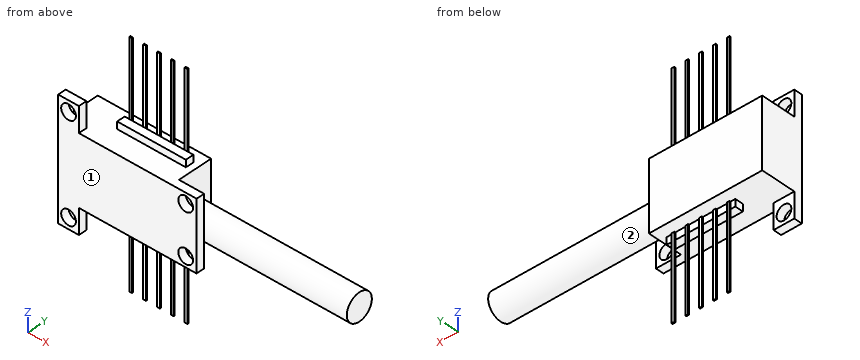
```python
from build123d import *

# Parameters (mm, degrees)
SKETCH1_W               = 20.8
SKETCH1_H               = 12.7
BOSS_EXTRUDE1_DEPTH     = 6.4
BOSS_EXTRUDE2_DEPTH     = 1.5
SKETCH5_R               = 1.35
CUT_EXTRUDE1_DEPTH      = 21.181984541
SKETCH8_R               = 2.5
BOSS_EXTRUDE3_DEPTH     = 30.15
SKETCH9_W               = 12.6
SKETCH9_H               = 1.3
BOSS_EXTRUDE4_DEPTH     = 1.5
SKETCH10_W              = 0.5
SKETCH10_H              = 15.3
BOSS_EXTRUDE5_DEPTH     = 0.2
LPATTERN1_COUNT         = 5
LPATTERN1_PITCH         = 2.54
MIRROR2_COPY_1_SKETCH_W = 0.5
MIRROR2_COPY_1_SKETCH_H = 15.3
MIRROR2_COPY_1_DEPTH    = 0.2
MIRROR2_COPY_2_SKETCH_W = 0.5
MIRROR2_COPY_2_SKETCH_H = 15.3
MIRROR2_COPY_2_DEPTH    = 0.2
MIRROR2_COPY_3_SKETCH_W = 0.5
MIRROR2_COPY_3_SKETCH_H = 15.3
MIRROR2_COPY_3_DEPTH    = 0.2
MIRROR2_COPY_4_SKETCH_W = 0.5
MIRROR2_COPY_4_SKETCH_H = 15.3
MIRROR2_COPY_4_DEPTH    = 0.2


with BuildPart() as part:
    # Sketch1 → Boss-Extrude1 (new body)
    with BuildSketch(Plane(origin=(0, 0, 0), x_dir=(1, 0, 0), z_dir=(0, 1, 0))):
        Rectangle(SKETCH1_W, SKETCH1_H)
    extrude(amount=BOSS_EXTRUDE1_DEPTH)

    # Sketch3 → Boss-Extrude2 (add)
    with BuildSketch(Plane.XZ):
        Polygon((-10.4, 10.95), (-6.6, 10.95), (-6.6, 6.35), (15, 6.35), (15, -6.35), (-6.6, -6.35), (-6.6, -10.95), (-10.4, -10.95), align=None)
    extrude(amount=BOSS_EXTRUDE2_DEPTH)

    # Sketch5 → Cut-Extrude1 (cut, through all)
    with BuildSketch(Plane.XZ.offset(1.5)):
        with Locations(Location((-8.5, 8.95, 0), (0, 0, 270))):
            Circle(SKETCH5_R)
        with Locations(Location((13, 4.45, 0), (0, 0, 270))):
            Circle(SKETCH5_R)
    cut_extrude1 = extrude(amount=-CUT_EXTRUDE1_DEPTH, mode=Mode.SUBTRACT)

    # Mirror3: Cut-Extrude1 across plane
    add(cut_extrude1.mirror(Plane.XY), mode=Mode.SUBTRACT)

    # Sketch8 → Boss-Extrude3 (add)
    with BuildSketch(Plane(origin=(10.4, 0, 0), x_dir=(0, 0, -1), z_dir=(1, 0, 0))):
        with Locations(Location((1.5, 3.2, 0), (0, 0, 180))):
            Circle(SKETCH8_R)
    extrude(amount=BOSS_EXTRUDE3_DEPTH)

    # Sketch9 → Boss-Extrude4 (add)
    with BuildSketch(Plane(origin=(0, 2.665, 0), x_dir=(-1, 0, 0), z_dir=(0, -1, 0))):
        with Locations((-2.9, -7)):
            Rectangle(SKETCH9_W, SKETCH9_H)
    boss_extrude4 = extrude(amount=-BOSS_EXTRUDE4_DEPTH)

    # Sketch10 → Boss-Extrude5 (add)
    with BuildSketch(Plane(origin=(0, 4.165, 0), x_dir=(1, 0, 0), z_dir=(0, 1, 0))):
        with Locations((7.87, -14)):
            Rectangle(SKETCH10_W, SKETCH10_H)
    boss_extrude5 = extrude(amount=BOSS_EXTRUDE5_DEPTH)

    # LPattern1: Boss-Extrude5 ×5
    with Locations(*[(-i * LPATTERN1_PITCH, 0, 0) for i in range(1, LPATTERN1_COUNT)]):
        add(boss_extrude5)

    # Mirror2: Boss-Extrude4, Boss-Extrude5 across plane
    add(boss_extrude4.mirror(Plane.XY))
    add(boss_extrude5.mirror(Plane.XY))

    # Mirror2 copy 1 sketch → Mirror2 copy 1 (add)
    with BuildSketch(Plane(origin=(-2.54, 4.165, 0), x_dir=(1, 0, 0), z_dir=(0, 1, 0))):
        with Locations((7.87, 14)):
            Rectangle(MIRROR2_COPY_1_SKETCH_W, MIRROR2_COPY_1_SKETCH_H)
    extrude(amount=MIRROR2_COPY_1_DEPTH)

    # Mirror2 copy 2 sketch → Mirror2 copy 2 (add)
    with BuildSketch(Plane(origin=(-5.08, 4.165, 0), x_dir=(1, 0, 0), z_dir=(0, 1, 0))):
        with Locations((7.87, 14)):
            Rectangle(MIRROR2_COPY_2_SKETCH_W, MIRROR2_COPY_2_SKETCH_H)
    extrude(amount=MIRROR2_COPY_2_DEPTH)

    # Mirror2 copy 3 sketch → Mirror2 copy 3 (add)
    with BuildSketch(Plane(origin=(-7.62, 4.165, 0), x_dir=(1, 0, 0), z_dir=(0, 1, 0))):
        with Locations((7.87, 14)):
            Rectangle(MIRROR2_COPY_3_SKETCH_W, MIRROR2_COPY_3_SKETCH_H)
    extrude(amount=MIRROR2_COPY_3_DEPTH)

    # Mirror2 copy 4 sketch → Mirror2 copy 4 (add)
    with BuildSketch(Plane(origin=(-10.16, 4.165, 0), x_dir=(1, 0, 0), z_dir=(0, 1, 0))):
        with Locations((7.87, 14)):
            Rectangle(MIRROR2_COPY_4_SKETCH_W, MIRROR2_COPY_4_SKETCH_H)
    extrude(amount=MIRROR2_COPY_4_DEPTH)


solid = part.part
```
Geometry: final body of the model. Coordinates: model frame, mm. Face numbers are marked on the shaded views. A direction names the side the tool comes from. Give positions to 0.01 mm unless a question says otherwise; leave off trailing zeros. Loops run counter-clockwise (first coordinate to the right, second up) from the corner with the lowest first, then second, coordinate; pieces in that order, holes last. Notation, with made-up numbers: (66, 74.25) -> (81, 74.25) arc R35 ccw to (81, 108.25) -> close; hole circle Ø5 at (46.5, -2.75). An arc over 180 degrees is marked (long way). Use one line per item in the form item = value.
Item 1: Section query D-D on x = -8.5. Output: boundary loops of the cut face in (y, z), and give its area (3 significant figures).
A:
outline = (-1.5, -10.95) -> (0, -10.95) -> (0, -10.3) -> (-1.5, -10.3) -> close; (-1.5, -7.6) -> (0, -7.6) -> (0, -6.35) -> (6.4, -6.35) -> (6.4, 6.35) -> (0, 6.35) -> (0, 7.6) -> (-1.5, 7.6) -> close; (-1.5, 10.3) -> (0, 10.3) -> (0, 10.95) -> (-1.5, 10.95) -> close
area = 106 mm^2
Item 2: Section query B-B on z = 4.45. Output: boundary loops of the cut face in (x, y), and give its area (3 significant figures).
A:
outline = (-10.4, -1.5) -> (11.65, -1.5) -> (11.65, 0) -> (10.4, 0) -> (10.4, 6.4) -> (-10.4, 6.4) -> close; (14.35, -1.5) -> (15, -1.5) -> (15, 0) -> (14.35, 0) -> close
area = 167 mm^2
Item 3: Access query for the marked faces 1 and 2. Directions: +Z, -Z, +X, -X, +Y, -Y. A direction counts if a zero-diameter tool reaches every point of the face in a straight line with its end or side. Return the directions, or none.
A:
face_1 = +Z, -Z, +X, -X, -Y
face_2 = +X
Item 4: Pin query (flat end, axial travel): P1, Ø0.6, axis at x = 5.5, z = 13, coming from the +Y side (3 decimals); P2, Ø3, axis at y = 3, z = -13, coming from the +X side; P3, Ø1.6, axis at y = -0.5, z = 8, coming from the +X side. Return the tip coordinate at first contact, or that it passes through.
A:
P1 = 4.365
P2 = 8.12
P3 = -6.6
Item 5: Line query: probe 1 along X at (y, z) = (-0.4, 8.95); probe 2 along X at (y, z) = (5.25, -4.5); probe 3 along X at (y, z) = (-0.7, 4.45). Output: solid intervals per line, ascending.
A:
probe_1 = -10.4 to -9.85, -7.15 to -6.6
probe_2 = -10.4 to 10.4
probe_3 = -10.4 to 11.65, 14.35 to 15
Item 6: Section query C-C on z = 15.5. Output: boundary loops of the cut face in (x, y) (3 decimals), and give its area (3 significant figures).
A:
outline = (-2.54, 4.165) -> (-2.04, 4.165) -> (-2.04, 4.365) -> (-2.54, 4.365) -> close; (0, 4.165) -> (0.5, 4.165) -> (0.5, 4.365) -> (0, 4.365) -> close; (2.54, 4.165) -> (3.04, 4.165) -> (3.04, 4.365) -> (2.54, 4.365) -> close; (5.08, 4.165) -> (5.58, 4.165) -> (5.58, 4.365) -> (5.08, 4.365) -> close; (7.62, 4.165) -> (8.12, 4.165) -> (8.12, 4.365) -> (7.62, 4.365) -> close
area = 0.500 mm^2
Item 7: Section query A-A on x = 13. Output: boundary loops of the cut face in (y, z).
A:
outline = (-1.5, -6.35) -> (0, -6.35) -> (0, -5.8) -> (-1.5, -5.8) -> close; (-1.5, -3.1) -> (0, -3.1) -> (0, 3.1) -> (-1.5, 3.1) -> close; (-1.5, 5.8) -> (0, 5.8) -> (0, 6.35) -> (-1.5, 6.35) -> close; circle Ø5 at (3.2, -1.5)
